```python
from build123d import *

# Parameters (mm, degrees)
F2_SIZE = 0.74999
F3_SIZE = 0.5


# Not quite as in the source:
# - a fillet or chamfer is up to 0.001 mm smaller than in the source, because OpenCascade refuses the exact size


with BuildPart() as f1:
    # F0 (on Front) → F1 (revolve)
    with BuildSketch(Plane.XZ):
        Polygon((-6, 0), (0, 0), (0, 106), (-5, 106), (-5, 87.5), (-4.25, 87.5), (-4.25, 86), (-5, 86), (-7.5, 86), (-7.5, 16), (-6, 16), (-6, 14.25), align=None)
    revolve(axis=Axis((0, 0, 53), (0, 0, -1)))

    # F2 (size 0.75 in the source; OpenCascade refuses exactly that, so slightly less here)
    f2_edges = [f1.edges().sort_by_distance(p)[0] for p in [
        (5, 0, 106),
        (5, 0, 87.5),
        (-5, 0, 96.75),
    ]]
    chamfer(f2_edges, length=F2_SIZE)

    # F3
    f3_edges = [f1.edges().sort_by_distance(p)[0] for p in [
        (7.5, 0, 86),
        (7.5, 0, 16),
        (-7.5, 0, 51),
        (6, 0, 0),
        (6, 0, 16),
    ]]
    chamfer(f3_edges, length=F3_SIZE)


solid = f1.part
```
Can you work these out from the model? Positions are in its coordinate system, mm. A direction names the side the tool comes from. Give positions to 0.01 mm unless a question says otherwise; leave off trailing zeros. Write each loop counter-clockwise with the first axis right and the second up, starting at its lowest first coordinate (ties: lowest second). Pieces come first, ordered by that corner, then holes. Notation, with made-up numbers: (18, -15) -> (24, -15) arc R15 cw to (24, 10) -> close; hole circle Ø8 at (-35, 56.25). An arc over 180 degrees is marked (long way). One line per item, written item: value.
Q1. Please list where these lines run through material, in increasing order: line 1 (Y direction, x = -0.5, z = 35.5); line 2 (Z direction, x = -6.5, y = -1.25); line 3 (Z direction, x = 0.75, y = -4.5). Write a range as [from, to].
Results found:
line 1: y = [-7.48, 7.48]
line 2: z = [16, 86]
line 3: z = [0, 86], [87.81, 105.69]
Q2. For P1, Ø1, axis at y = -5, z = 12, coming from the +X side; P2, Ø8, axis at y = -4.5, z = 84, coming from the +X side; P3, Ø2, axis at y = -3.5, z = 64, coming from the +X side, each with a flat end and sliding along its axis, tell me the tip position at first contact or that it passes through.
Results found:
P1: stops at x = 3.97
P2: stops at x = 7.48
P3: stops at x = 7.07
Q3. Which directions (+Z, -Z, +X, -X, +Y, -Y) give clear straight access to the entire face, cutting with the end or side of a thin tool? Please do faces 1 (the face through (1.08, -4.88, 96.63)), 2 (the face through (0, 0, 0)), 3 (the face through (6, 0, 8)), 4 (the face through (0, -5, 86)).
Results found:
face 1: +Z
face 2: -Z, +X, -X, +Y, -Y
face 3: -Z
face 4: none
Q4. Imagine slicing it at C-C on z = 73. Please give me the cut outline in (x, y).
Results found:
outline: circle Ø15 at (0, 0)
